from build123d import *

# Parameters (mm, degrees)
SKETCH1_W           = 63.5
SKETCH1_H           = 95.25
SKETCH1_W_2         = 57.15
SKETCH1_H_2         = 88.9
EXTRUDE_THIN1_DEPTH = 25.4
FILLET1_R           = 3.175
BOSS_EXTRUDE1_DEPTH = 3.175
FILLET2_R           = 3.175
SKETCH3_R           = 2.06375
CUT_EXTRUDE1_DEPTH  = 3.175
CIRPATTERN1_COUNT   = 2
FILLET3_R           = 1.5875


with BuildPart() as part:
    # Sketch1 → Extrude-Thin1 (new body)
    with BuildSketch(Plane(origin=(0, 0, 0), x_dir=(1, 0, 0), z_dir=(0, 1, 0))):
        Rectangle(SKETCH1_W, SKETCH1_H)
        Rectangle(SKETCH1_W_2, SKETCH1_H_2, mode=Mode.SUBTRACT)
    extrude(amount=EXTRUDE_THIN1_DEPTH)

    # Fillet1
    fillet1_edges = [part.edges().sort_by_distance(p)[0] for p in [
        (28.575, 12.7, 44.45),
        (28.575, 12.7, -44.45),
        (-28.575, 12.7, -44.45),
        (-28.575, 12.7, 44.45),
        (31.75, 12.7, 47.625),
        (-31.75, 12.7, 47.625),
        (-31.75, 12.7, -47.625),
        (31.75, 12.7, -47.625),
    ]]
    fillet(fillet1_edges, radius=FILLET1_R)

    # Sketch2 → Boss-Extrude1 (add)
    with BuildSketch(Plane.XZ):
        with BuildLine():
            Line((31.75, -44.45), (31.75, 44.45))
            ThreePointArc((31.75, 44.45), (30.82006403, 46.69506403), (28.575, 47.625))
            Line((28.575, 47.625), (-28.575, 47.625))
            ThreePointArc((-28.575, 47.625), (-30.82006403, 46.69506403), (-31.75, 44.45))
            Line((-31.75, 44.45), (-31.75, -44.45))
            ThreePointArc((-31.75, -44.45), (-30.82006403, -46.69506403), (-28.575, -47.625))
            Line((-28.575, -47.625), (28.575, -47.625))
            ThreePointArc((28.575, -47.625), (30.82006403, -46.69506403), (31.75, -44.45))
        make_face()
    extrude(amount=BOSS_EXTRUDE1_DEPTH)

    # Fillet2
    fillet2_edges = [part.edges().sort_by_distance(p)[0] for p in [
        (28.575, 0, 0),
        (0, 0, -44.45),
        (-28.575, 0, 0),
        (0, 0, 44.45),
        (-27.64506403, 0, 43.52006403),
        (27.64506403, 0, 43.52006403),
        (27.64506403, 0, -43.52006403),
        (-27.64506403, 0, -43.52006403),
    ]]
    fillet(fillet2_edges, radius=FILLET2_R)

    # Sketch3 → Cut-Extrude1 (cut)
    with BuildSketch(Plane(origin=(0, 0, 0), x_dir=(1, 0, 0), z_dir=(0, 1, 0))):
        with Locations(Location((-19.05, 34.925, 0), (0, 0, 270))):
            Circle(SKETCH3_R)
    cut_extrude1 = extrude(amount=-CUT_EXTRUDE1_DEPTH, mode=Mode.SUBTRACT)

    # Sketch4 → Cut-Revolve1 (revolve, cut)
    with BuildSketch(Plane.YX.offset(34.925), mode=Mode.PRIVATE) as cut_revolve1_sk:
        Polygon((-2.480052205, -19.05), (0, -14.9225), (0, -19.05), align=None)
    cut_revolve1 = revolve(cut_revolve1_sk.sketch.rotate(Axis((-19.05, 0, -34.925), (0, -1, 0)), 90), axis=Axis((-19.05, 0, -34.925), (0, -1, 0)), mode=Mode.SUBTRACT)

    # CirPattern1: Cut-Extrude1, Cut-Revolve1 ×2 about axis
    cirpattern1_axis = Axis((0, 0, 0), (0, 1, 0))
    add([cut_extrude1.rotate(cirpattern1_axis, i * 360 / CIRPATTERN1_COUNT) for i in range(1, CIRPATTERN1_COUNT)], mode=Mode.SUBTRACT)
    add([cut_revolve1.rotate(cirpattern1_axis, i * 360 / CIRPATTERN1_COUNT) for i in range(1, CIRPATTERN1_COUNT)], mode=Mode.SUBTRACT)

    # Fillet3
    fillet3_edges = [part.edges().sort_by_distance(p)[0] for p in [
        (31.75, 25.4, 0),
        (0, 25.4, 47.625),
        (0, 25.4, -47.625),
        (-31.75, 25.4, 0),
        (0, 25.4, -44.45),
        (28.575, 25.4, 0),
        (0, 25.4, 44.45),
        (-28.575, 25.4, 0),
        (-30.82006403, 25.4, 46.69506403),
        (30.82006403, 25.4, -46.69506403),
        (-30.82006403, 25.4, -46.69506403),
        (30.82006403, 25.4, 46.69506403),
        (-27.64506403, 25.4, 43.52006403),
        (27.64506403, 25.4, 43.52006403),
        (27.64506403, 25.4, -43.52006403),
        (-27.64506403, 25.4, -43.52006403),
    ]]
    fillet(fillet3_edges, radius=FILLET3_R - 0.0001)  # a hair under: the kernel refuses the full size


solid = part.part
The listing builds one solid part. Answer for the finished solid, in the listing's coordinates (mm). A direction names the side the tool comes from. Coordinates: 2 decimals unless noted, no trailing zeros. Write each loop counter-clockwise with the first axis right and the second up, starting at its lowest first coordinate (ties: lowest second). Pieces come first, ordered by that corner, then holes. Notation, with made-up numbers: (11, 49) -> (61, 49) arc R14 cw to (61, 68) -> close; hole circle Ø3 at (34.5, 0.5). An arc over 180 degrees is marked (long way). One line per question, with ' | ' between items.
1. For a pull along X with two mould halves and no side action, classify faces 1 (the flat face through (28.575, 13, 1)), 2 (the flat face through (0, -3.175, 1)) as released by +X, released by -X, zero draft, split by the parting line, or undercut.
Verdict:
face 1: undercut | face 2: zero draft
2. Which of the six approach directions +Z, -Z, +X, -X, +Y, -Y give full straight-line access (tool end or side, diameter ignored) to faces 3 (the cylindrical face through (-27.67, 0.955, 0.578)), 4 (the cylindrical face through (19.84, -2.19, 33.02))?
Verdict:
face 3: +Y | face 4: +Y, -Y
3. Straight lines are drawn through the part: line 1 (X direction, y = 21.5, z = 12) (3 decimals); line 2 (Z direction, x = 19.05, y = -2.1) (3 decimals); line 3 (Z direction, x = 25.5, y = 16) (3 decimals). For each, find the intervals that lie inside material, in ascending order.
Verdict:
line 1: x = -31.75 to -28.575, 28.575 to 31.75 | line 2: z = -47.625 to 32.861, 36.989 to 47.625 | line 3: z = -47.625 to -44.448, 44.448 to 47.625
4. Section A-A (y = 21) is taken. Determine the outline of the cut face in (x, z) (3 decimals), and give its area (3 significant figures).
Verdict:
outline: (-31.75, -44.45) arc R3.175 ccw to (-28.575, -47.625) -> (28.575, -47.625) arc R3.175 ccw to (31.75, -44.45) -> (31.75, 44.45) arc R3.175 ccw to (28.575, 47.625) -> (-28.575, 47.625) arc R3.175 ccw to (-31.75, 44.45) -> close; hole (-28.575, -41.275) arc R3.175 ccw to (-25.4, -44.45) -> (25.4, -44.45) arc R3.175 ccw to (28.575, -41.275) -> (28.575, 41.275) arc R3.175 ccw to (25.4, 44.45) -> (-25.4, 44.45) arc R3.175 ccw to (-28.575, 41.275) -> close | area: 968 mm^2
5. Given pin 1 Ø1.5 at (x, z) = (-15, 28.5) entering from +Y; pin 2 Ø6.5 at (x, z) = (19.05, 34.925) entering from +Y, each flat-ended and moving along its own axis, determine where each tip first touches the part or whether it passes through.
Verdict:
pin 1: stops at y = 0 | pin 2: stops at y = -0.53
